Verification items for the finished model (mm, model axes). A direction names the side the tool comes from. Give positions to 0.01 mm unless a question says otherwise; leave off trailing zeros. Order: outer loops, then holes, each group sorted by start corner. A loop starts at its lowest first (then second) coordinate and runs counter-clockwise, first axis right, second up.
from build123d import *

# Parameters (mm, degrees)
SKETCH1_R           = 6.15
BOSS_EXTRUDE1_DEPTH = 28.575
SKETCH3_W           = 25.4
SKETCH3_H           = 12.7
BOSS_EXTRUDE2_DEPTH = 9.325


with BuildPart() as part:
    # Sketch1 → Boss-Extrude1 (new body)
    with BuildSketch(Plane(origin=(0, 0, 0), x_dir=(1, 0, 0), z_dir=(0, 1, 0))):
        with Locations(Location((0, 1.507106584, 0), (0, 0, 270))):
            Circle(SKETCH1_R)
    extrude(amount=BOSS_EXTRUDE1_DEPTH)

    # Sketch3 → Boss-Extrude2 (add)
    with BuildSketch(Plane(origin=(0, 28.575, 0), x_dir=(1, 0, 0), z_dir=(0, 1, 0))):
        with Locations((0, 1.507106584)):
            Rectangle(SKETCH3_W, SKETCH3_H)
    extrude(amount=BOSS_EXTRUDE2_DEPTH)

    # Chamfer1
    # the kernel refuses this chamfer: 1.5875 mm, written as the material it takes off along each edge
    with BuildSketch(Plane(origin=(-11.641666667, 29.633333333, -6.798773251), x_dir=(0.7071067811865478, -0.707106781186547, 0), z_dir=(-0.5773502691896255, -0.5773502691896262, -0.5773502691896257))) as chamfer1_piece_1:
        Polygon((-1.122532015, 0.648094161), (1.122532015, 0.648094161), (0, -1.296188322), align=None)
    extrude(amount=2.016395815, mode=Mode.SUBTRACT)
    with BuildSketch(Plane(origin=(-12.7, 28.575, 8.925440159), x_dir=(-0.027495876610586785, 0.9996219169112966, 0), z_dir=(0, 0, -1))) as chamfer1_piece_2:
        with BuildLine():
            Line((1.633018697, 0), (-0.089768608, 1.630549497))
            Line((-0.089768608, 1.630549497), (-0.121506604, 1.629676503))
            ThreePointArc((-0.121506604, 1.629676503), (-0.054180148, 0.815019055), (-0.031737996, -0.000872994))
            Line((-0.031737996, -0.000872994), (0.000872994, -0.031737996))
            ThreePointArc((0.000872994, -0.031737996), (0.816765043, -0.009295844), (1.633891691, -0.031737996))
            Line((1.633891691, -0.031737996), (1.633018697, 0))
        make_face()
    extrude(amount=20.865093487, mode=Mode.SUBTRACT)
    with BuildSketch(Plane(origin=(-12.7, 24.492453257, -7.857106584), x_dir=(-0.02749587661058674, 0, 0.9996219169112966), z_dir=(0, 1, 0))) as chamfer1_piece_3:
        with BuildLine():
            Line((1.633018697, 0), (-0.089768608, 1.630549497))
            Line((-0.089768608, 1.630549497), (-0.121506604, 1.629676503))
            ThreePointArc((-0.121506604, 1.629676503), (-0.054180148, 0.815019055), (-0.031737996, -0.000872994))
            Line((-0.031737996, -0.000872994), (0.000872994, -0.031737996))
            ThreePointArc((0.000872994, -0.031737996), (0.816765043, -0.009295844), (1.633891691, -0.031737996))
            Line((1.633891691, -0.031737996), (1.633018697, 0))
        make_face()
    extrude(amount=17.490093487, mode=Mode.SUBTRACT)
    with BuildSketch(Plane(origin=(16.782546743, 28.575, 4.842893416), x_dir=(0, 0.9996219169112966, 0.02749587661058624), z_dir=(-1, 0, 0))) as chamfer1_piece_4_section:
        with BuildLine():
            Line((1.633018697, 0), (-0.089768608, 1.630549497))
            Line((-0.089768608, 1.630549497), (-0.121506604, 1.629676503))
            ThreePointArc((-0.121506604, 1.629676503), (-0.054180148, 0.815019055), (-0.031737996, -0.000872994))
            Line((-0.031737996, -0.000872994), (0.000872994, -0.031737996))
            ThreePointArc((0.000872994, -0.031737996), (0.816765043, -0.009295844), (1.633891691, -0.031737996))
            Line((1.633891691, -0.031737996), (1.633018697, 0))
        make_face()
    chamfer1_piece_4 = extrude(amount=33.565093487, mode=Mode.PRIVATE)
    chamfer1_piece_4 = chamfer1_piece_4 - Plane(origin=(0, 29.903258734, -1.507106584), x_dir=(0, 0, 1), z_dir=(0, -1, 0)) * Cylinder(6.15, 74, mode=Mode.PRIVATE)
    add(chamfer1_piece_4, mode=Mode.SUBTRACT)
    with BuildSketch(Plane(origin=(12.7, 24.492453257, 4.842893416), x_dir=(-0.9996219169112968, 0, 0.027495876610586185), z_dir=(0, 1, 0)), Plane(origin=(12.7, 24.492453257, -7.857106584), x_dir=(0.027495876610586754, 0, 0.9996219169112966), z_dir=(0, 1, 0))) as chamfer1_piece_5:
        with BuildLine():
            Line((1.633018697, 0), (-0.089768608, -1.630549497))
            Line((-0.089768608, -1.630549497), (-0.121506604, -1.629676503))
            ThreePointArc((-0.121506604, -1.629676503), (-0.054180148, -0.815019055), (-0.031737996, 0.000872994))
            Line((-0.031737996, 0.000872994), (0.000872994, 0.031737996))
            ThreePointArc((0.000872994, 0.031737996), (0.816765043, 0.009295844), (1.633891691, 0.031737996))
            Line((1.633891691, 0.031737996), (1.633018697, 0))
        make_face()
    extrude(amount=17.490093487, mode=Mode.SUBTRACT)
    with BuildSketch(Plane(origin=(-16.782546743, 28.575, -7.857106584), x_dir=(0, -0.027495876610585654, 0.9996219169112968), z_dir=(1, 0, 0))) as chamfer1_piece_6_section:
        with BuildLine():
            Line((1.633018697, 0), (-0.089768608, -1.630549497))
            Line((-0.089768608, -1.630549497), (-0.121506604, -1.629676503))
            ThreePointArc((-0.121506604, -1.629676503), (-0.054180148, -0.815019055), (-0.031737996, 0.000872994))
            Line((-0.031737996, 0.000872994), (0.000872994, 0.031737996))
            ThreePointArc((0.000872994, 0.031737996), (0.816765043, 0.009295844), (1.633891691, 0.031737996))
            Line((1.633891691, 0.031737996), (1.633018697, 0))
        make_face()
    chamfer1_piece_6 = extrude(amount=33.565093487, mode=Mode.PRIVATE)
    chamfer1_piece_6 = chamfer1_piece_6 - Plane(origin=(0, 28.785057027, -1.507106584), x_dir=(0, 0, 1), z_dir=(0, -1, 0)) * Cylinder(6.15, 74, mode=Mode.PRIVATE)
    add(chamfer1_piece_6, mode=Mode.SUBTRACT)


solid = part.part
(1) Go/stop test with flat-tipped pins: pin 1 (2 mm diameter, centred on y = 28, z = -3.5, fed in from -X); pin 2 (4 mm diameter, centred on y = 9, z = 3.5, fed in from -X); pin 3 (4 mm diameter, centred on y = 19.5, z = -3.5, fed in from -X). Record where each tip stops, or that it passes through.
Solved:
pin 1: stops at x = -11.54
pin 2: stops at x = -5.36
pin 3: stops at x = -6.15
(2) Scan lines: line 1 (Y direction, x = -6.5, z = 2.25) (3 decimals); line 2 (Y direction, x = -10.75, z = 3.5); line 3 (Z direction, x = 4, y = 12). Record each from-to range of solid material in increasing order.
Solved:
line 1: y = 28.575 to 37.9
line 2: y = 28.82 to 37.9
line 3: z = -6.18 to 3.16
(3) Section check B-B, the plane z = -1. Enter the section's corners in (x, y) (1 decimal), then the cut area to 3 significant figures.
Solved:
outline: (-12.7, 30.2) - (-11.1, 28.6) - (-6.1, 28.6) - (-6.1, 0) - (6.1, 0) - (6.1, 28.6) - (12.7, 28.6) - (12.7, 37.9) - (-12.7, 37.9) - close
area: 586 mm2
(4) Section check C-C, the plane y = 18.5. Enter the section's corners in (x, z).
Solved:
outline: circle Ø12.3 at (0, -1.51)
(5) Section check A-A, the plane x = -2.25. Enter the section's corners in (y, z), then the cut area to 3 significant figures.
Solved:
outline: (0, -7.23) - (29.54, -7.23) - (30.16, -7.86) - (37.9, -7.86) - (37.9, 4.84) - (30.16, 4.84) - (29.54, 4.22) - (0, 4.22) - close
area: 444 mm2
(6) Section check D-D, the plane x = 5. Enter the section's corners in (y, z) (1 decimal), then the cut area to 3 significant figures.
Solved:
outline: (0, -5.1) - (28.6, -5.1) - (28.6, -6.3) - (30.2, -7.9) - (37.9, -7.9) - (37.9, 4.8) - (30.2, 4.8) - (28.6, 3.3) - (28.6, 2.1) - (0, 2.1) - close
area: 321 mm2
(7) Set-up check for faces 1 (the flat face through (-2.64, 29.56, 4.24)), 2 (the flat face through (3.273, 29.358, -7.052)), 3 (the cylindrical face through (-1.516, 14.876, 4.453)): record each of +Z, -Z, +X, -X, +Y, -Y from which the full face is reachable in a straight line by a thin tool's end or side.
Solved:
face 1: +Z, -Y
face 2: -Z, -Y
face 3: -Y
